Input: part model. Units: mm. Frame: model coordinates. Face numbers are marked on the shaded views. A direction names the side the tool comes from. Give positions to 0.01 mm unless a question says otherwise; leave off trailing zeros. Loops run counter-clockwise (first coordinate to the right, second up) from the corner with the lowest first, then second, coordinate; pieces in that order, holes last. Notation, with made-up numbers: M 18.5,89.25 L 59.5,89.25 A25 cw 59.5,110.25 Z; hole C 22,11 d6. An arc over 180 degrees is marked long. Use a Markdown table: item, result. Add a question column.
from build123d import *

# Parameters (mm, degrees)
SKETCH1_W           = 175
SKETCH1_H           = 6.75
BOSS_EXTRUDE1_DEPTH = 6.5
SKETCH2_W           = 10
SKETCH2_H           = 6.75
BOSS_EXTRUDE2_DEPTH = 7.5
SKETCH5_R           = 3.175
CUT_EXTRUDE2_DEPTH  = 10
LPATTERN1_COUNT     = 6
LPATTERN1_PITCH     = 25
SKETCH6_R           = 3.175
BOSS_EXTRUDE4_DEPTH = 6.75
LPATTERN2_COUNT     = 6
LPATTERN2_PITCH     = 25
BOSS_EXTRUDE5_DEPTH = 6.5
BOSS_EXTRUDE6_DEPTH = 3
SKETCH10_R          = 2.55
CUT_EXTRUDE4_DEPTH  = 2
CUT_EXTRUDE5_DEPTH  = 18


with BuildPart() as part:
    # Sketch1 → Boss-Extrude1 (new body)
    with BuildSketch(Plane(origin=(0, 0, 0), x_dir=(1, 0, 0), z_dir=(0, 1, 0))):
        with Locations((87.5, -3.375)):
            Rectangle(SKETCH1_W, SKETCH1_H)
    extrude(amount=BOSS_EXTRUDE1_DEPTH)

    # Sketch2 → Boss-Extrude2 (add)
    with BuildSketch(Plane(origin=(0, 6.5, 0), x_dir=(1, 0, 0), z_dir=(0, 1, 0))):
        with Locations((5, -3.375)):
            Rectangle(SKETCH2_W, SKETCH2_H)
    boss_extrude2 = extrude(amount=BOSS_EXTRUDE2_DEPTH)

    # Sketch5 → Cut-Extrude2 (cut)
    with BuildSketch(Plane.XY.offset(6.75)):
        with Locations((5, 8.75)):
            Circle(SKETCH5_R)
    cut_extrude2 = extrude(amount=-CUT_EXTRUDE2_DEPTH, mode=Mode.SUBTRACT)

    # LPattern1: Boss-Extrude2, Cut-Extrude2 ×6
    with Locations(*[(i * LPATTERN1_PITCH, 0, 0) for i in range(1, LPATTERN1_COUNT)]):
        add(boss_extrude2)
        add(cut_extrude2, mode=Mode.SUBTRACT)

    # Sketch6 → Boss-Extrude4 (add)
    with BuildSketch(Plane.XY.offset(6.75)):
        Polygon((138.660254038, 8.75), (138.660254038, 0), (121.339745962, 0), (121.339745962, 8.75), (125.669872981, 16.25), (134.330127019, 16.25), align=None)
        with Locations((130, 8.75)):
            Circle(SKETCH6_R, mode=Mode.SUBTRACT)
    boss_extrude4 = extrude(amount=-BOSS_EXTRUDE4_DEPTH)

    # LPattern2: Boss-Extrude4 ×6
    with Locations(*[(-i * LPATTERN2_PITCH, 0, 0) for i in range(1, LPATTERN2_COUNT)]):
        add(boss_extrude4)

    # Sketch7 → Boss-Extrude5 (add)
    with BuildSketch(Plane(origin=(0, 6.5, 0), x_dir=(1, 0, 0), z_dir=(0, 1, 0))):
        Polygon((172.113248654, -8.375), (177.886751346, -8.375), (178.824945533, -6.75), (182.289047149, -6.75), (179.618802154, -11.375), (170.381197846, -11.375), (165.762395693, -3.375), (170.381197846, 4.625), (179.618802154, 4.625), (181.350852961, 1.625), (177.886751346, 1.625), (172.113248654, 1.625), (169.226497308, -3.375), align=None)
    extrude(amount=-BOSS_EXTRUDE5_DEPTH)

    # Sketch9 → Boss-Extrude6 (add)
    with BuildSketch(Plane(origin=(0, 0, 0), x_dir=(-1, 0, 0), z_dir=(0, -1, 0))):
        Polygon((-169.226497308, -3.375), (-172.113248654, 1.625), (-177.886751346, 1.625), (-181.350852961, 1.625), (-184.237604307, -3.375), (-182.289047149, -6.75), (-178.824945533, -6.75), (-177.886751346, -8.375), (-172.113248654, -8.375), align=None)
    extrude(amount=-BOSS_EXTRUDE6_DEPTH)

    # Sketch10 → Cut-Extrude4 (cut)
    with BuildSketch(Plane(origin=(0, 0, 0), x_dir=(-1, 0, 0), z_dir=(0, -1, 0))):
        with Locations((-175, -3.375)):
            Circle(SKETCH10_R)
    extrude(amount=-CUT_EXTRUDE4_DEPTH, mode=Mode.SUBTRACT)

    # Sketch11 → Cut-Extrude5 (cut)
    with BuildSketch(Plane(origin=(0, 3, 0), x_dir=(1, 0, 0), z_dir=(0, 1, 0))):
        Polygon((180.773502692, -3.375), (177.886751346, 1.625), (172.113248654, 1.625), (169.226497308, -3.375), (172.113248654, -8.375), (177.886751346, -8.375), align=None)
    extrude(amount=CUT_EXTRUDE5_DEPTH, mode=Mode.SUBTRACT)


solid = part.part
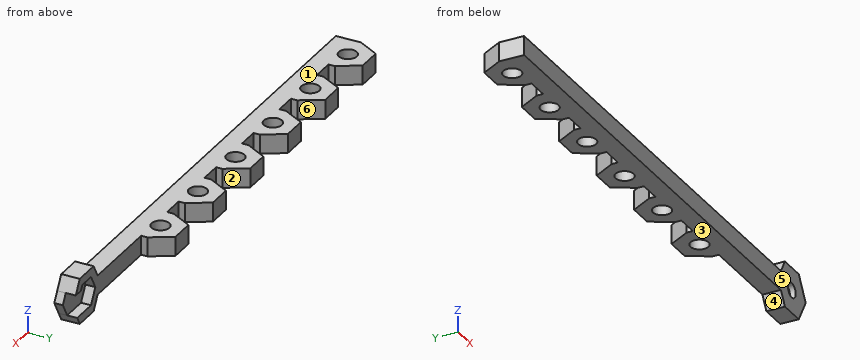
1) Section query D-D, the plane x = 154. Return the cut outline in (y, z), and give its area (3 significant figures).
2) Ray query, line 1 (Z direction, x = 174, y = 6) (3 decimals); line 2 (Y direction, x = 130, z = 3) (3 decimals); line 3 (Z direction, x = 175, y = 0.8) (3 decimals). Return the intervals inside material, ascending. Write a range as [from, to].
3) Section query C-C, the plane x = 81.5. Return the cut outline in (y, z).
4) Pull-direction query (X, two-part tool) for the marked faces 4, 5 and 6; classes: pulls with the +X half, pulls with the -X half, needs draft (parallel to the pull), parting line crosses it, or undercut.
5) Reachability of the marked faces 1, 2 and 3 from +Z, -Z, +X, -X, +Y, -Y: full face, straight path, thin tool, end or side. Return the list, or none.
6) Section query B-B, the plane x = 175. Return the cut outline in (y, z) (3 decimals).
7) Section query A-A, the plane x = 30. Return the cut outline in (y, z) (3 decimals).
8) Contact query for flat-ended pins moving along their axis: P1, Ø5.5, axis at x = 42.5, z = 1.5, coming from the +Y side; P2, Ø5, axis at x = 56, y = 8.5, coming from the +Z side; P3, Ø4, axis at x = 105, y = 8.75, coming from the +Z side; P4, Ø1.1, axis at y = 7.5, z = 2.5, coming from the +X side. Output: stop coordinate, or through.
Entries:
| question | item | result |
|---|---|---|
| 1 | outline | M 0,0 L 6.5,0 L 6.5,6.75 L 0,6.75 Z |
| 1 | area | 43.9 mm² |
| 2 | line 1 | z = [-4.625, -1.625], [8.375, 11.375] |
| 2 | line 2 | y = [0, 5.575], [11.925, 16.25] |
| 2 | line 3 | z = [-4.625, 0.825], [5.925, 11.375] |
| 3 | outline | M 0,0 L 5.95,0 L 5.95,6.75 L 0,6.75 Z; M 11.55,0 L 16.25,0 L 16.25,6.75 L 11.55,6.75 Z |
| 4 | face 4 | pulls with the -X half |
| 4 | face 5 | needs draft |
| 4 | face 6 | undercut |
| 5 | face 1 | +Z, -X, +Y, -Y |
| 5 | face 2 | +Z, -Z, +Y |
| 5 | face 3 | -Z, -X, +Y, -Y |
| 6 | outline | M 0,-4.625 L 6.5,-4.625 L 6.5,-1.625 L 3,-1.625 L 3,8.375 L 6.5,8.375 L 6.5,11.375 L 0,11.375 L 0,5.925 L 2,5.925 L 2,0.825 L 0,0.825 Z |
| 7 | outline | M 0,0 L 5.575,0 L 5.575,6.75 L 0,6.75 Z; M 11.925,0 L 16.25,0 L 16.25,6.75 L 11.925,6.75 Z |
| 8 | P1 | stops at y = 6.5 |
| 8 | P2 | stops at z = 6.75 |
| 8 | P3 | passes through |
| 8 | P4 | stops at x = 138.66 |
